Could you check a few things on this drawing? It's one solid part, dimensions in mm from its lowest x, y, z. A direction names the side the tool comes from. Coordinates: 2 decimals unless noted, no trailing zeros. Order: outer loops, then holes, each group sorted by start corner. A loop starts at its lowest first (then second) coordinate and runs counter-clockwise, first axis right, second up. Notation, with made-up numbers: (-31.75, 44.25) - (16.25, 44.25) arc R21 cw to (16.25, 62.25) - close; hole circle Ø10 at (82.25, 47.25). An arc over 180 degrees is marked (long way). Answer in a Markdown table with one row per item. Add a question column.
Item 1: If I drill on line 1 along X through (y, z) = (77.5, 32); line 2 along X through (y, z) = (37.5, 11.5); line 3 along Y through (x, z) = (74.5, 2), over which ranges is the centre line in solid material (lowest first)? Write a range as from..to.
Item 2: I want a section at D-D (x = 74). Please give me the cut outline in (y, z).
Item 3: I want a section at A-A (x = 50). Please give me the cut outline in (y, z), plus the area to 3 significant figures.
Item 4: On a 3-axis mill with a long thin cutter (end or side, diameter ignored), from which of +Z, -Z, +X, -X, +Y, -Y can I reach the whole of each face in a straight line? I mean the marked faces 4, 5 and 6. Say none if no direction works.
Item 5: Will these pins go through, and if not, where does the flat tip stop? pin 1 Ø4 at (x, z) = (35, 14.5) entering from +Y; pin 2 Ø5 at (x, z) = (47.5, 6.5) entering from +Y; pin 3 Ø3 at (y, z) = (37.5, 13) entering from -X.
Item 6: I want a section at B-B (y = 61). Please give me the cut outline in (x, z).
Item 7: Thinking about a two-plate mould opening in Y: for the marked faces 1, 2 and 3, which applies, +Y half, -Y half, draft (parallel to the pull), parting line (faces both ways), or undercut?
Item 8: I want a section at C-C (z = 29). Please give me the cut outline in (x, y), plus the area to 3 significant figures.
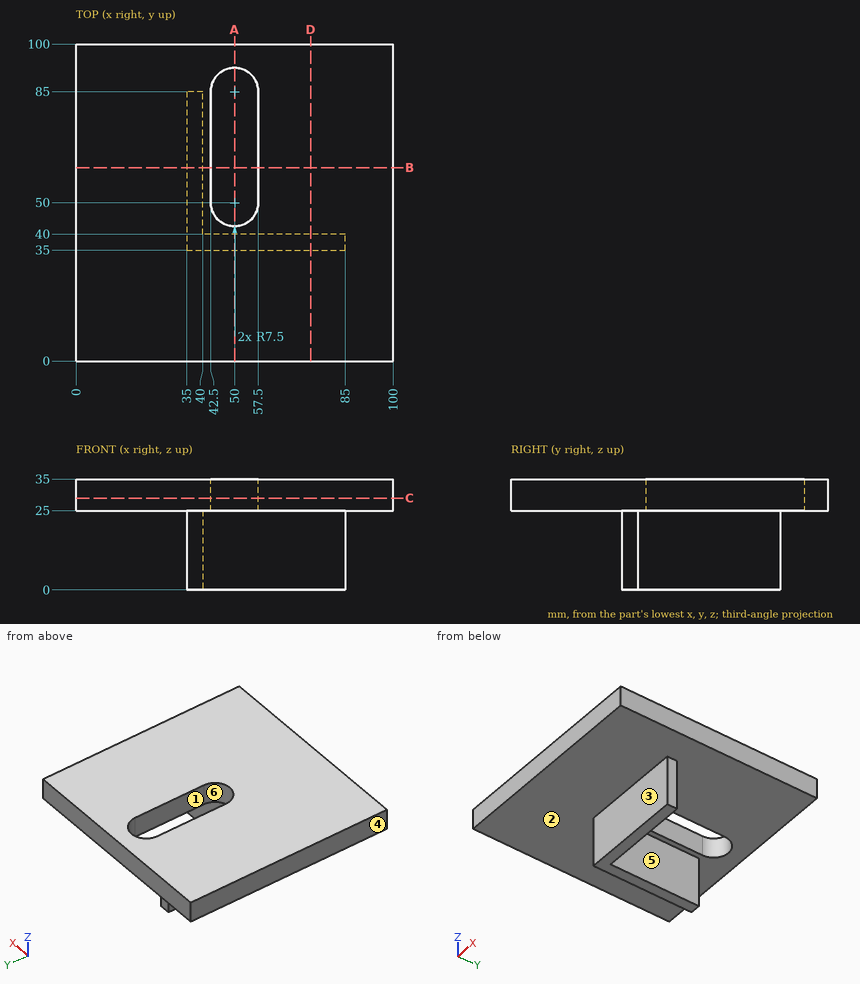
Values follow:
| question | item | result |
|---|---|---|
| 1 | line 1 | x = 0..42.5, 57.5..100 |
| 1 | line 2 | x = 35..85 |
| 1 | line 3 | y = 35..40 |
| 2 | outline | (0, 25) - (35, 25) - (35, 0) - (40, 0) - (40, 25) - (100, 25) - (100, 35) - (0, 35) - close |
| 3 | outline | (0, 25) - (35, 25) - (35, 0) - (40, 0) - (40, 25) - (42.5, 25) - (42.5, 35) - (0, 35) - close; (92.5, 25) - (100, 25) - (100, 35) - (92.5, 35) - close |
| 3 | area | 625 mm^2 |
| 4 | face 4 | +Z, -Z, -X, +Y, -Y |
| 4 | face 5 | -Z, +X, +Y |
| 4 | face 6 | +Z, -Z |
| 5 | pin 1 | stops at y = 85 |
| 5 | pin 2 | stops at y = 40 |
| 5 | pin 3 | stops at x = 35 |
| 6 | outline | (0, 25) - (35, 25) - (35, 0) - (40, 0) - (40, 25) - (42.5, 25) - (42.5, 35) - (0, 35) - close; (57.5, 25) - (100, 25) - (100, 35) - (57.5, 35) - close |
| 7 | face 1 | undercut |
| 7 | face 2 | draft |
| 7 | face 3 | -Y half |
| 8 | outline | (0, 0) - (100, 0) - (100, 100) - (0, 100) - close; hole (42.5, 50) arc R7.5 ccw to (57.5, 50) - (57.5, 85) arc R7.5 ccw to (42.5, 85) - close |
| 8 | area | 9,300 mm^2 |
